Source: CAD feature listing. Evaluate the final solid. Frame: model axes, mm. Face numbers are marked on the shaded views. A direction names the side the tool comes from. Round coordinates to 2 decimals unless told otherwise and drop trailing zeros. Order: outer loops, then holes, each group sorted by start corner. A loop starts at its lowest first (then second) coordinate and runs counter-clockwise, first axis right, second up. Notation, with made-up numbers: M -38,71 L -12,71 A13 ccw -12,81 Z; hole C 60,26 d9. An arc over 180 degrees is marked long. Answer in a Markdown table with one row per item. Add a question column.
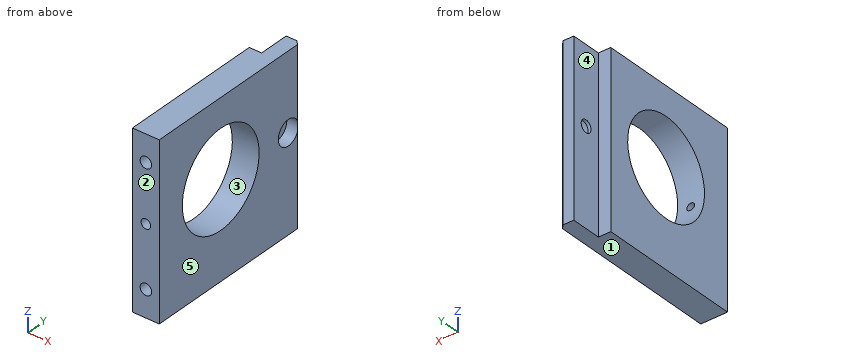
```python
from build123d import *

# Parameters (mm, degrees)
BOSS_EXTRUDE1_DEPTH            = 45
CBORE_FOR_M3_SHCS1_D           = 3.2
CBORE_FOR_M3_SHCS1_CBORE_D     = 6.5
CBORE_FOR_M3_SHCS1_CBORE_DEPTH = 3
F_25_0_25_DIAMETER_HOLE1_D     = 25
CHAMFER1_SIZE                  = 1
F_3_0MM_DOWEL_HOLE1_D          = 3
F_3_0MM_DOWEL_HOLE1_DEPTH      = 4.5
F_3_0MM_DOWEL_HOLE1_TIP        = 0.901290929
M3X0_5_TAPPED_HOLE1_D          = 2.5
M3X0_5_TAPPED_HOLE1_DEPTH      = 7.5
M3X0_5_TAPPED_HOLE1_TIP        = 0.751075774


with BuildPart() as part:
    # Sketch1 → Boss-Extrude1 (new body)
    with BuildSketch(Plane.XY):
        Polygon((3.23, 30.362745098), (3.23, 22.362745098), (0, 22.362745098), (0, -15.637254902), (7, -15.637254902), (7, 30.362745098), align=None)
    extrude(amount=BOSS_EXTRUDE1_DEPTH)

    # CBORE for M3 SHCS1 (through all)
    with Locations(Plane(origin=(7, 0, 0), x_dir=(0, 0, -1), z_dir=(1, 0, 0))):
        with Locations((-25, 26.362745098)):
            CounterBoreHole(CBORE_FOR_M3_SHCS1_D / 2, CBORE_FOR_M3_SHCS1_CBORE_D / 2, CBORE_FOR_M3_SHCS1_CBORE_DEPTH)

    # Ø25.0 (25) Diameter Hole1 (through all)
    with Locations(Plane(origin=(7, 0, 0), x_dir=(0, 0, -1), z_dir=(1, 0, 0))):
        with Locations((-25, 4.362745098)):
            Hole(F_25_0_25_DIAMETER_HOLE1_D / 2)

    # Chamfer1
    # the kernel refuses this chamfer: 1 mm, written as the material it takes off along each edge
    with BuildSketch(Plane(origin=(7, 30.362745098, -2.571682988), x_dir=(-0.9996219169112968, 0.027495876610585623, 0), z_dir=(0, 0, 1))) as chamfer1_piece_1:
        Polygon((CHAMFER1_SIZE * 0.999621916911, CHAMFER1_SIZE * 0.0274958766106), (-CHAMFER1_SIZE * 0.0274958766106, CHAMFER1_SIZE * 0.999621916911), (0, 0), align=None)
    extrude(amount=50.143365976, mode=Mode.SUBTRACT)

    # Ø3.0mm Dowel Hole1
    with Locations(Plane(origin=(0, -15.637254902, 0), x_dir=(-1, 0, 0), z_dir=(0, -1, 0))):
        with Locations((-3.5, -38), (-3.5, -7)):
            Hole(F_3_0MM_DOWEL_HOLE1_D / 2, depth=F_3_0MM_DOWEL_HOLE1_DEPTH)
            with Locations((0, 0, -(F_3_0MM_DOWEL_HOLE1_DEPTH + F_3_0MM_DOWEL_HOLE1_TIP / 2))):  # 118° drill point
                Cone(0, F_3_0MM_DOWEL_HOLE1_D / 2, F_3_0MM_DOWEL_HOLE1_TIP, mode=Mode.SUBTRACT)

    # M3x0.5 Tapped Hole1
    with Locations(Plane(origin=(0, -15.637254902, 0), x_dir=(-1, 0, 0), z_dir=(0, -1, 0))):
        with Locations((-3.5, -23)):
            Hole(M3X0_5_TAPPED_HOLE1_D / 2, depth=M3X0_5_TAPPED_HOLE1_DEPTH)
            with Locations((0, 0, -(M3X0_5_TAPPED_HOLE1_DEPTH + M3X0_5_TAPPED_HOLE1_TIP / 2))):  # 118° drill point
                Cone(0, M3X0_5_TAPPED_HOLE1_D / 2, M3X0_5_TAPPED_HOLE1_TIP, mode=Mode.SUBTRACT)


solid = part.part
```
(1) Cut plane B-B (y = 16). Return loops of the section in (x, z).
(2) Pin query (flat end, axial travel): pin 1 (9 mm diameter, centred on y = 27, z = 22, fed in from -X); pin 2 (2.5 mm diameter, centred on x = 3.5, z = 38, fed in from -Y); pin 3 (2 mm diameter, centred on y = -0.5, z = 6.5, fed in from -X); pin 4 (3.5 mm diameter, centred on y = 26.36, z = 25, fed in from +X). Return the tip coordinate at first contact, or that it passes through.
(3) Line query: line 1 (Z direction, x = 3.5, y = -9.25); line 2 (Y direction, x = 5, z = 27.5); line 3 (X direction, y = -12.9, z = 7). Output: solid intervals per line, ascending. Write a range as from..to.
(4) Cut plane A-A (z = 25). Return loops of the section in (x, y).
(5) Cut plane D-D (y = 5). Return loops of the section in (x, z).
(6) Access query for the marked faces 4 and 5. Directions: +Z, -Z, +X, -X, +Y, -Y. A direction counts if a zero-diameter tool reaches every point of the face in a straight line with its end or side. Return the directions, or none.
(7) Draft query along Y for the marked faces 1, 2 and 3. Return one class per face: +Y half, -Y half, draft (parallel to the pull), parting line (faces both ways), or undercut.
(8) Cut plane C-C (z = 17.5). Return loops of the section in (x, y), and give its area (3 significant figures).
Answer list:
| question | item | result |
|---|---|---|
| 1 | outline | M 0,0 L 7,0 L 7,20.44 L 0,20.44 Z; M 0,29.56 L 7,29.56 L 7,45 L 0,45 Z |
| 2 | pin 1 | x = 3.23 |
| 2 | pin 2 | y = -10.99 |
| 2 | pin 3 | x = 0 |
| 2 | pin 4 | x = 4 |
| 3 | line 1 | 0..21.75, 24.25..45 |
| 3 | line 2 | -15.64..-7.88, 16.61..24.29, 28.44..30.36 |
| 3 | line 3 | 0..2, 5..7 |
| 4 | outline | M 0,-15.64 L 7,-15.64 L 7,-8.14 L 0,-8.14 Z; M 0,16.86 L 7,16.86 L 7,23.11 L 4,23.11 L 4,24.76 L 3.23,24.76 L 3.23,22.36 L 0,22.36 Z; M 3.23,27.96 L 4,27.96 L 4,29.61 L 6.75,29.61 L 6,30.36 L 3.23,30.36 Z |
| 5 | outline | M 0,0 L 7,0 L 7,12.52 L 0,12.52 Z; M 0,37.48 L 7,37.48 L 7,45 L 0,45 Z |
| 6 | face 4 | +Z, -Z, -X, +Y |
| 6 | face 5 | +Z, -Z, +X, +Y, -Y |
| 7 | face 1 | draft |
| 7 | face 2 | -Y half |
| 7 | face 3 | undercut |
| 8 | outline | M 0,-15.64 L 7,-15.64 L 7,-5.64 L 0,-5.64 Z; M 0,14.36 L 7,14.36 L 7,29.36 L 6,30.36 L 3.23,30.36 L 3.23,22.36 L 0,22.36 Z |
| 8 | area | 156 mm² |
